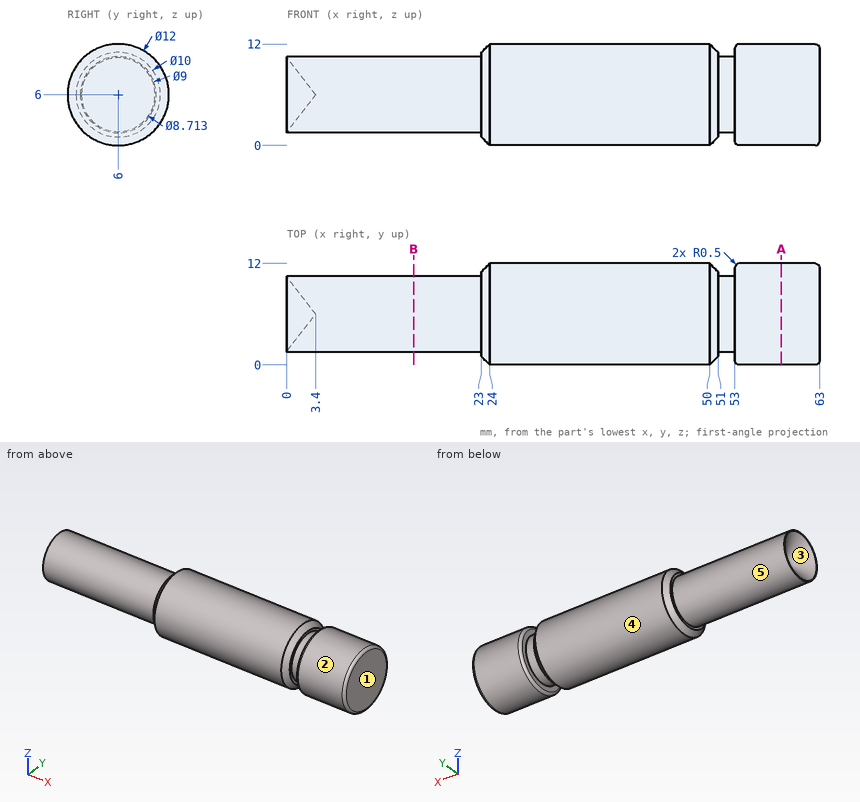
Verification items for this drawing (mm, ordinates from the low corner). A direction names the side the tool comes from. Round coordinates to 2 decimals unless told otherwise and drop trailing zeros. Loops run counter-clockwise (first coordinate to the right, second up) from the corner with the lowest first, then second, coordinate; pieces in that order, holes last. Notation, with made-up numbers: M 77,68 L 126,68 A28 ccw 126,90 Z; hole C -34,-22 d1. An arc over 180 degrees is marked long. Answer as a JSON object with one key per item and string values.
1. Section check B-B (x = 15). Record the boundary of the cut face in (y, z), plus the area to 3 significant figures.
Reply:
{"outline": "C 6,6 d9", "area": "63.6 mm²"}
2. Mould release check, pull along Y, two halves, no side actions. Record for the marked faces 1, 2 and 3: pulls with the +Y half, pulls with the -Y half, needs draft (parallel to the pull), parting line crosses it, or undercut.
Reply:
{"face 1": "needs draft", "face 2": "parting line crosses it", "face 3": "undercut"}
3. Gauge pin test, flat ends, axial feed: P1, Ø6, axis at x = 31, y = 4.5, coming from the +Z side; P2, Ø4, axis at x = 18, y = 3.5, coming from the +Z side; P3, Ø4, axis at x = 28, y = 9, coming from the -Z side; P4, Ø1, axis at x = 20, z = 10.5, coming from the -Y side. Record the tip position at first contact, or that the pin passes through.
Reply:
{"P1": "stops at z = 12", "P2": "stops at z = 10.47", "P3": "stops at z = 0.08", "P4": "stops at y = 3.94"}
4. Access from +Z, -Z, +X, -X, +Y, -Y to the whole of each face (thin tool, end or side, straight path). Record for the marked faces 4 and 5.
Reply:
{"face 4": "+X, -X", "face 5": "-X"}
5. Section check A-A (x = 58.5). Record the boundary of the cut face in (y, z).
Reply:
{"outline": "C 6,6 d12"}
6. Scan lines: line 1 (X direction, y = 9, z = 9.5); line 2 (Z direction, x = 7.5, y = 6); line 3 (X direction, y = 10.5, z = 8.5). Record each from-to range of solid material in increasing order.
Reply:
{"line 1": "x = 23 to 51, 53 to 63", "line 2": "z = 1.5 to 10.5", "line 3": "x = 23.15 to 50.85, 53 to 63"}
